Solid Edge part; units mm, degrees
sketch "Sketch1" plane through (0, 0, 0) normal (0, 0, 1) x (1, 0, 0)
  line L0 (2.0207, -3.5) -> (-2.0207, -3.5)
  line L1 (-4.0415, 0) -> (-2.0207, -3.5)
  line L2 (-2.0207, 3.5) -> (-4.0415, 0)
  line L3 (-2.0207, 3.5) -> (2.0207, 3.5)
  line L4 (2.0207, 3.5) -> (4.0415, 0)
  line L5 (4.0415, 0) -> (2.0207, -3.5)
extrude "Protrusion1" add sketch "Sketch1" along normal mid plane 3
sketch "Sketch2" plane through (0, 0, 0) normal (1, 0, 0) x (0, 1, 0)
  line L0 (-3.5, 1.5) -> (-1.7635, 3.2365)
revolve "RevolvedCutout1" cut sketch "Sketch2" angle 360 about axis through (0, 0, -57) along (0, 0, 1) material side at (0, -2.6671, 2.4036)
mirror "Mirror1" about plane through (0, 0, 0) normal (0, 0, 1) of "RevolvedCutout1"
sketch "Sketch3" plane through (0, 0, 0) normal (1, 0, 0) x (0, 1, 0)
  line L0 (0, 1.5) -> (0, 3.5)
  line L1 (0, 3.5) -> (-2.5, 3.5)
  arc A0 (-3.5, 2.5) -> (-2.5, 3.5) centre (-2.5, 2.5) cw
  line L2 (-3.5, 2.5) -> (-3.5, 1.5)
  line L3 (-3.5, 1.5) -> (0, 1.5)
revolve "RevolvedProtrusion1" add sketch "Sketch3" angle 360 about axis through (0, 0, -57) along (0, 0, 1)
hole "Hole_1" at (0, 0, 1.5) direction (0, 0, 1) diameter 3.242 end through all both ways yes
sketch "Sketch4" plane through (0, 0, 3.5) normal (0, 0, 1) x (0, 1, 0)
  circle A0 centre (0, 0) radius 2.25
extrude "ExtrudedCutout_1" cut sketch "Sketch4" against normal blind 1
sketch "Sketch5" plane through (0, 0, 0) normal (1, 0, 0) x (0, 1, 0)
  line L0 (-2.25, 2.5) -> (-1.45, 2.5)
  line L1 (-1.45, 2.5) -> (-1.45, 3.5)
  line L2 (-1.45, 3.5) -> (-2.25, 3.5)
  line L3 (-2.25, 3.5) -> (-2.25, 2.5)
revolve "RevolvedProtrusion2" add sketch "Sketch5" angle 360 about axis through (0, 0, -57) along (0, 0, 1)
Geometry: final body of the model. Coordinates: model frame, mm. Round coordinates to 2 decimals unless told otherwise and drop trailing zeros. Write each loop counter-clockwise with the first axis right and the second up, starting at its lowest first coordinate (ties: lowest second). Pieces come first, ordered by that corner, then holes. Notation, with made-up numbers: (-27.75, -34.75) -> (-7.75, -34.75) arc R24 ccw to (-7.75, 4.25) -> close; hole circle Ø5 at (-2, 79.5). An arc over 180 degrees is marked (long way). Return JSON: item names as keys, results as strings.
Q1. Mould query, pull axis X, two halves, no side actions, for faces 1 (the cylindrical face through (0.06, 1.45, 3.01)), 2 (the conical face through (3.7, -0.1, -1.3)), 3 (the flat face through (0, 3.5, 0)), 4 (the cylindrical face through (1.341, -3.233, 1.993)). Classes: +X half, -X half, draft (parallel to the pull), parting line (faces both ways), or undercut.
From the geometry:
{"face 1": "undercut", "face 2": "+X half", "face 3": "draft", "face 4": "parting line"}
Q2. Section A-A on z = -0.3. Return the cut outline in (x, y), and give its area (3 significant figures).
From the geometry:
{"outline": "(-4.04, 0) -> (-2.02, -3.5) -> (2.02, -3.5) -> (4.04, 0) -> (2.02, 3.5) -> (-2.02, 3.5) -> close; hole circle Ø3.24 at (0, 0)", "area": "34.2 mm2"}
Q3. Section B-B on z = 1.2. Return the cut outline in (x, y), and give its area (3 significant figures).
From the geometry:
{"outline": "(-3.77, -0.47) -> (-2.29, -3.03) arc R3.8 ccw to (-1.48, -3.5) -> (1.48, -3.5) arc R3.8 ccw to (2.29, -3.03) -> (3.77, -0.47) arc R3.8 ccw to (3.77, 0.47) -> (2.29, 3.03) arc R3.8 ccw to (1.48, 3.5) -> (-1.48, 3.5) arc R3.8 ccw to (-2.29, 3.03) -> (-3.77, 0.47) arc R3.8 ccw to start; hole circle Ø3.24 at (0, 0)", "area": "33.5 mm2"}
Q4. First-contact query: pin 1 Ø1.6 at (x, y) = (0.5, 0.5) entering from -Z. Flat tip, straight axial feed; report the tip coordinate or a pass-through.
From the geometry:
{"pin 1": "z = 2.5"}
Q5. Ray query, line 1 (X direction, y = 0, z = 1.8); line 2 (X direction, y = -1, z = 0.3); line 3 (Y direction, x = -0.5, z = 1.65). Return the intervals inside material, ascending.
From the geometry:
{"line 1": "-3.5 to -1.62, 1.62 to 3.5", "line 2": "-3.46 to -1.28, 1.28 to 3.46", "line 3": "-3.46 to -1.54, 1.54 to 3.46"}
Q6. Section C-C on z = 2. Return the cut outline in (x, y).
From the geometry:
{"outline": "circle Ø7 at (0, 0); hole circle Ø3.24 at (0, 0)"}
